Geometry: final body of the model. Coordinates: model frame, mm. Round coordinates to 2 decimals unless told otherwise and drop trailing zeros. Loops run counter-clockwise (first coordinate to the right, second up) from the corner with the lowest first, then second, coordinate; pieces in that order, holes last. Notation, with made-up numbers: M -14,6 L 33,6 A30 ccw 33,44 Z; hole C -19.5,42.5 d7. An arc over 180 degrees is marked long. Return JSON: item names as keys, results as strings.
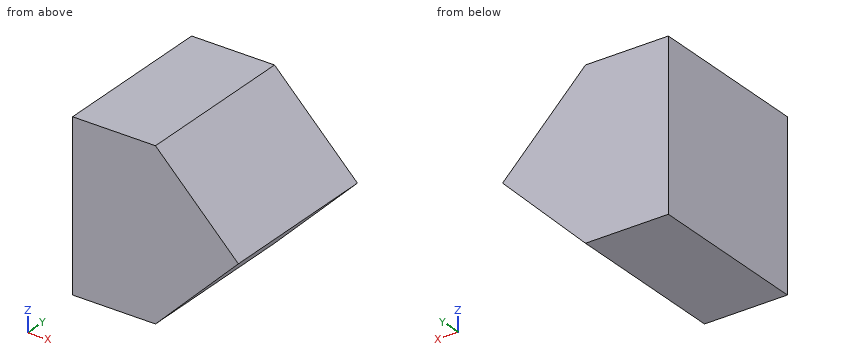
from build123d import *

# Parameters (mm, degrees)
SKETCH1_W           = 20
SKETCH1_H           = 20
BOSS_EXTRUDE1_DEPTH = 20
CUT_EXTRUDE1_DEPTH  = 20
CUT_EXTRUDE2_DEPTH  = 20


with BuildPart() as part:
    # Sketch1 → Boss-Extrude1 (new body)
    with BuildSketch(Plane.XY):
        with Locations((10, 10)):
            Rectangle(SKETCH1_W, SKETCH1_H)
    extrude(amount=BOSS_EXTRUDE1_DEPTH)

    # Sketch2 → Cut-Extrude1 (cut)
    with BuildSketch(Plane(origin=(0, 20, 0), x_dir=(1, 0, 0), z_dir=(0, 1, 0))):
        Polygon((20, 0), (10, 0), (20, -10), align=None)
    extrude(amount=-CUT_EXTRUDE1_DEPTH, mode=Mode.SUBTRACT)

    # Sketch3 → Cut-Extrude2 (cut)
    with BuildSketch(Plane(origin=(0, 20, 0), x_dir=(1, 0, 0), z_dir=(0, 1, 0))):
        Polygon((20, -20), (10, -20), (20, -10), align=None)
    extrude(amount=-CUT_EXTRUDE2_DEPTH, mode=Mode.SUBTRACT)


solid = part.part
Q1. Pin query (flat end, axial travel): pin 1 (4 mm diameter, centred on y = 5.5, z = 16.5, fed in from +X); pin 2 (3 mm diameter, centred on y = 9, z = 7.5, fed in from -X); pin 3 (4 mm diameter, centred on y = 2.5, z = 14, fed in from +X); pin 4 (1 mm diameter, centred on y = 2, z = 2.5, fed in from +X). Return the tip coordinate at first contact, or that it passes through.
Determined:
{"pin 1": "stops at x = 15.5", "pin 2": "stops at x = 0", "pin 3": "stops at x = 18", "pin 4": "stops at x = 13"}
Q2. Section query B-B (z = 6.75). Output: boundary loops of the cut face in (x, y).
Determined:
{"outline": "M 0,0 L 16.75,0 L 16.75,20 L 0,20 Z"}
Q3. Section query A-A (y = 7). Output: boundary loops of the cut face in (x, z).
Determined:
{"outline": "M 0,0 L 10,0 L 20,10 L 10,20 L 0,20 Z"}
Q4. Section query C-C (x = 12). Output: boundary loops of the cut face in (y, z), plus the area to 3 significant figures.
Determined:
{"outline": "M 0,2 L 20,2 L 20,18 L 0,18 Z", "area": "320 mm^2"}
Q5. Material intervals for L1, parallel to X at y = 8, z = 5.25; L2, parallel to X at y = 9, z = 19.25; L3, parallel to Z at x = 16.25, y = 3.75, sorted ascending.
Determined:
{"L1": "x = 0 to 15.25", "L2": "x = 0 to 10.75", "L3": "z = 6.25 to 13.75"}
